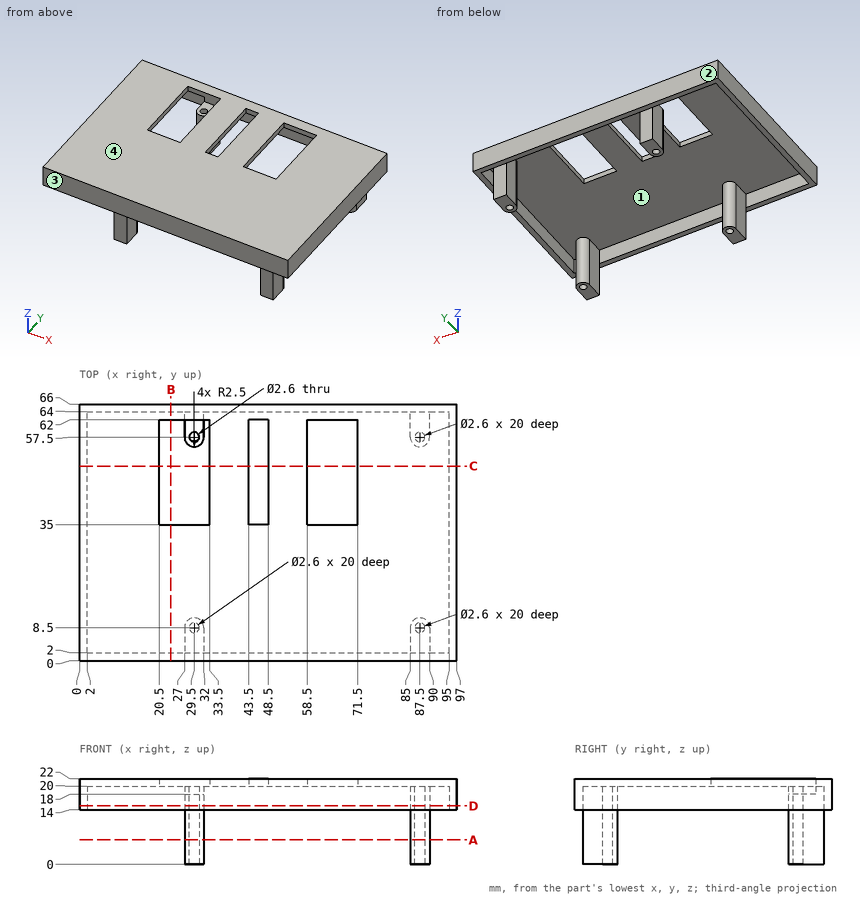
Check sheet for the drawn part. Datum: minimum x, y, z corner. Units: mm. Give positions to 0.01 mm unless a question says otherwise; leave off trailing zeros. Order: outer loops, then holes, each group sorted by start corner. A loop starts at its lowest first (then second) coordinate and runs counter-clockwise, first axis right, second up.
1. Sectioned sample at D-D (z = 15). Record the boundary of the cut face in (x, y).
Completed:
outline: (0, 0) - (97, 0) - (97, 66) - (0, 66) - close; hole (2, 2) - (27, 2) - (27, 8.5) arc R2.5 cw to (32, 8.5) - (32, 2) - (85, 2) - (85, 8.5) arc R2.5 cw to (90, 8.5) - (90, 2) - (95, 2) - (95, 64) - (90, 64) - (90, 57.5) arc R2.5 cw to (85, 57.5) - (85, 64) - (32, 64) - (32, 57.5) arc R2.5 cw to (27, 57.5) - (27, 64) - (2, 64) - close; hole circle Ø2.6 at (29.5, 8.5); hole circle Ø2.6 at (29.5, 57.5); hole circle Ø2.6 at (87.5, 8.5); hole circle Ø2.6 at (87.5, 57.5)
2. Sectioned sample at C-C (y = 50). Record the boundary of the cut face in (x, z).
Completed:
outline: (0, 14) - (2, 14) - (2, 20) - (20.5, 20) - (20.5, 22) - (0, 22) - close; (33.5, 20) - (43.5, 20) - (43.5, 22) - (33.5, 22) - close; (48.5, 20) - (58.5, 20) - (58.5, 22) - (48.5, 22) - close; (71.5, 20) - (95, 20) - (95, 14) - (97, 14) - (97, 22) - (71.5, 22) - close
3. Depth check by flat-ended pin: pin 1 (8 mm diameter, centred on x = 39, z = 3, fed in from -Y); pin 2 (8 mm diameter, centred on x = 83, z = 9, fed in from +Y); pin 3 (1.5 mm diameter, centred on x = 35.5, y = 56, fed in from -Z); pin 4 (1.5 mm diameter, centred on x = 30, y = 59, fed in from +Z). Enter the tip coordinate at first touch or a pass-through.
Completed:
pin 1: passes through
pin 2: stops at y = 64
pin 3: stops at z = 20
pin 4: stops at z = 18
4. Scan lines: line 1 (Y direction, x = 29.5, z = 13); line 2 (X direction, y = 42, z = 19.75); line 3 (Z direction, x = 40, y = 57). Record each from-to range of solid material in increasing order.
Completed:
line 1: y = 2 to 7.2, 9.8 to 11, 55 to 56.2, 58.8 to 64
line 2: x = 0 to 2, 95 to 97
line 3: z = 20 to 22
5. Sectioned sample at A-A (z = 6.25). Record the boundary of the cut face in (x, y), then the cut area to 3 significant figures.
Completed:
outline: (27, 2) - (32, 2) - (32, 8.5) arc R2.5 ccw to (27, 8.5) - close; (27, 57.5) arc R2.5 ccw to (32, 57.5) - (32, 64) - (27, 64) - close; (85, 2) - (90, 2) - (90, 8.5) arc R2.5 ccw to (85, 8.5) - close; (85, 57.5) arc R2.5 ccw to (90, 57.5) - (90, 64) - (85, 64) - close; hole circle Ø2.6 at (29.5, 8.5); hole circle Ø2.6 at (29.5, 57.5); hole circle Ø2.6 at (87.5, 8.5); hole circle Ø2.6 at (87.5, 57.5)
area: 148 mm2
6. Sectioned sample at B-B (x = 23.5). Record the boundary of the cut face in (y, z), then the cut area to 3 significant figures.
Completed:
outline: (0, 14) - (2, 14) - (2, 20) - (35, 20) - (35, 22) - (0, 22) - close; (62, 20) - (64, 20) - (64, 14) - (66, 14) - (66, 22) - (62, 22) - close
area: 102 mm2
7. Draft check along Y on the marked faces 1, 2, 3 and 4. Enter one of: pulls with the +Y half, pulls with the -Y half, needs draft (parallel to the pull), parting line crosses it, or undercut.
Completed:
face 1: undercut
face 2: pulls with the +Y half
face 3: pulls with the -Y half
face 4: needs draft
